CAD build for the part. Positions are in the model's coordinates, mm. A direction names the side the tool comes from. Round coordinates to 2 decimals unless told otherwise and drop trailing zeros. Order: outer loops, then holes, each group sorted by start corner. A loop starts at its lowest first (then second) coordinate and runs counter-clockwise, first axis right, second up. Notation, with made-up numbers: (19.25, 61) -> (23.25, 61) arc R15 ccw to (23.25, 66) -> close; hole circle Ø4 at (-8.75, -38.5). An arc over 180 degrees is marked (long way). Answer as CSV lines item,"result". Start each with the question number.
Autodesk Inventor part; units mm, degrees
ref_plane "YZ Plane" through (0, 0, 0) normal (1, 0, 0) x (0, 1, 0)
ref_plane "XZ Plane" through (0, 0, 0) normal (0, 1, 0) x (-1, 0, 0)
ref_plane "XY Plane" through (0, 0, 0) normal (0, 0, 1) x (1, 0, 0)
sketch "Sketch1" plane through (0, 0, 0) normal (0, 0, 1) x (1, 0, 0)
  circle A0 centre (0, 0) radius 1.75
  circle A1 centre (0, 0) radius 3.5
  circle A2 centre (0, 0) radius 5.75 construction
  line L0 (0, 0) -> (0, 5.75) construction
  circle A3 centre (0.5, 9.2365) radius 3.5
  line L1 (0, 0) -> (0, 5.75) construction
  line L2 (3.5, 0) -> (3.5, 5.75)
  line L3 (-3.5, 5.75) -> (-3.5, 0)
  arc A4 (-3.5, 0) -> (3.5, 0) centre (0, 0) ccw
  arc A5 (3.5, 5.75) -> (-1.9961, 2.875) centre (0, 5.75) ccw
  arc A6 (-3.4062, 0.805) -> (-3.4062, 4.945) centre (-12.1649, 2.875) ccw
  line L4 (0.5, 5.7365) -> (3.5, 5.7365)
  point P0 (0, 2.875)
  point P1 (-3.4345, 6.424)
  point P2 (3.5, 0)
  point P3 (3.244, 7.0639)
  point P4 (-3.5, 0)
  point P5 (-2.744, 7.9226)
  dimension "d2" = 11.5
  dimension "d3" = 7
  dimension "d0" = 3.5
  dimension "d1" = 7
  dimension "d4" = 3.5
  dimension "d9" = 0.5
  dimension "d10" = 9
extrude "Extrusion1" add sketch "Sketch1" along normal blind 4.7625 contours A1 | A1 A5 A3 L4 L2 | A1 A6 A5 | L3 A5 A6 A1
fillet "Fillet1" radius 1 1 edges at (-2.744, 7.9226, 2.3813)
fillet "Fillet2" radius 2 1 edges at (3.5, 5.7365, 2.3813)
sketch "Sketch2" plane through (0, 0, 0) normal (0, 0, -1) x (-1, 0, 0)
  line L0 (-3.5, 0) -> (-3.5, 3.7365)
  arc A0 (-3.5, 0) -> (3.5, 0) centre (0, 0) ccw
  circle A1 centre (0, 0) radius 1.75
  circle A2 centre (0, 0) radius 6.0263 construction
  arc A3 (3.4953, 5.9311) -> (1.8307, 6.6254) centre (2.4966, 5.8794) ccw
  arc A4 (-0.5, 5.7365) -> (1.8307, 6.6254) centre (-0.5, 9.2365) ccw
  line L1 (3.5, 5.75) -> (3.5, 0)
  line L2 (-1.5, 5.7365) -> (-0.5, 5.7365)
  arc A5 (-1.5, 5.7365) -> (-3.5, 3.7365) centre (-1.5, 3.7365) ccw
  arc A6 (-1.5, 5.7365) -> (-3.5, 3.7365) centre (-1.5, 3.7365) ccw
  arc A7 (3.5, 5.75) -> (3.4953, 5.9311) centre (0, 5.75) ccw
equation "\"d4\" = 0.5 * d1"
properties part number "Cam - Lever" material "Nylon 6/6"
Item 1: Band-saw the part on A-A, the plane y = -0.5. Give the cut face in (x, z).
Item 2: Band-saw the part on B-B, the plane x = -1.5. Give the cut face in (y, z), and give its area (3 significant figures).
Item 3: Mould opens along X. For faces 3 (the cylindrical face through (0.1, -3.5, 2.3)), 4 (the flat face through (0, 2, 0)), 5 (the cylindrical face through (-0.73, 5.96, 2.35)), 6 (the cylindrical face through (1.617, 0.67, 2.348)) say: released by +X, released by -X, zero draft, split by the parting line, or undercut.
Item 4: Tool access for faces 1 (the flat face through (3.5, 2, 2)), 2 (the flat face through (1, 5.736, 2)): list every direction of +Z, -Z, +X, -X, +Y, -Y with a clear straight run to the whole face (end or side of a thin tool).
Item 5: Band-saw the part on C-C, the plane y = -2. Give the cut face in (x, z), and give its area (3 significant figures).
Item 6: Probe line 1 (Y direction, x = 0, z = 2.55); line 2 (Y direction, x = -1.5, z = 3.2); line 3 (X direction, y = -0.25, z = 2.15). List the from-to ranges inside material, lowest first.
Values:
1,outline,"(-3.46, 0) -> (-1.68, 0) -> (-1.68, 4.76) -> (-3.46, 4.76) -> close; (1.68, 0) -> (3.46, 0) -> (3.46, 4.76) -> (1.68, 4.76) -> close"
2,outline,"(-3.16, 0) -> (-0.9, 0) -> (-0.9, 4.76) -> (-3.16, 4.76) -> close; (0.9, 0) -> (6.36, 0) -> (6.36, 4.76) -> (0.9, 4.76) -> close"
2,area,"36.8 mm²"
3,face 3,"split by the parting line"
3,face 4,"zero draft"
3,face 5,"released by +X"
3,face 6,"undercut"
4,face 1,"+Z, -Z, +X, +Y, -Y"
4,face 2,"+Z, -Z, +X, +Y"
5,outline,"(-2.87, 0) -> (2.87, 0) -> (2.87, 4.76) -> (-2.87, 4.76) -> close"
5,area,"27.4 mm²"
6,line 1,"-3.5 to -1.75, 1.75 to 5.77"
6,line 2,"-3.16 to -0.9, 0.9 to 6.36"
6,line 3,"-3.49 to -1.73, 1.73 to 3.49"
